```python
from build123d import *

# Parameters (mm, degrees)
F1_DEPTH = 3.175
F3_DEPTH = 12.7
F5_DEPTH = 12.7


with BuildPart() as f1:
    # F0 (on Top) → F1 (new body)
    with BuildSketch(Plane.XY):
        Polygon((-6.0333638393, 76.2), (-12.7, 0), (12.7, 0), (6.0333638393, 76.2), align=None)
    extrude(amount=-F1_DEPTH)

    # F2 (on face) → F3 (join)
    with BuildSketch(Plane.XY):
        Polygon((-2.8583638393, 76.2), (-6.0333638393, 76.2), (-12.7, 0), (-9.525, 0), align=None)
        Polygon((12.7, 0), (6.0333638393, 76.2), (2.8583638393, 76.2), (9.525, 0), align=None)
    extrude(amount=F3_DEPTH)

    # F4 (on face) → F5 (cut, through all)
    with BuildSketch(Plane.XY.offset(12.7)):
        Polygon((0, 15.875), (-11.3111174665, 15.875), (-12.4222234933, 3.175), (0, 3.175), align=None)
    extrude(amount=-F5_DEPTH, mode=Mode.SUBTRACT)


solid = f1.part
```
Build history of the part. All positions in model axes, mm. A direction names the side the tool comes from. Coordinates: 2 decimals unless noted, no trailing zeros. Write each loop counter-clockwise with the first axis right and the second up, starting at its lowest first coordinate (ties: lowest second). Pieces come first, ordered by that corner, then holes.
1. Band-saw the part on B-B, the plane y = 68.5. Give the cut face in (x, z) (3 decimals), and give its area (3 significant figures).
Answer block:
outline: (-6.707, -3.175) - (6.707, -3.175) - (6.707, 12.7) - (3.532, 12.7) - (3.532, 0) - (-3.532, 0) - (-3.532, 12.7) - (-6.707, 12.7) - close
area: 123 mm2
2. Band-saw the part on D-D, the plane z = -2. Give the cut face in (x, y), and give its area (3 significant figures).
Answer block:
outline: (-12.7, 0) - (12.7, 0) - (6.03, 76.2) - (-6.03, 76.2) - close
area: 1,430 mm2
3. Drop flat-ended pins along their axis: pin 1 (5 mm diameter, centred on y = 59.5, z = 5.5, fed in from -X); pin 2 (5 mm diameter, centred on x = -1.5, y = 22.5, fed in from +Z); pin 3 (5 mm diameter, centred on y = 66, z = 0.5, fed in from +X). Give the stop position or say it passes through.
Answer block:
pin 1: stops at x = -7.71
pin 2: stops at z = 0
pin 3: stops at x = 7.14
4. Drill centre lines: probe 1 along Z at (x, y) = (1.5, 64.5) (3 decimals); probe 2 along X at (y, z) = (55, 5); probe 3 along X at (y, z) = (68.5, 2.25). Where is each one in solid material? Low to high.
Answer block:
probe 1: z = -3.175 to 0
probe 2: x = -7.89 to -4.71, 4.71 to 7.89
probe 3: x = -6.71 to -3.53, 3.53 to 6.71
5. Pull direction Y, two halves, no side cores. Call faces 4 (the flat face through (-10, 15.875, 6)), 5 (the flat face through (0, 0, -1)), 6 (the flat face through (0, 30, -3.175)): released by +Y, released by -Y, zero draft, split by the parting line, or undercut.
Answer block:
face 4: undercut
face 5: released by -Y
face 6: zero draft
6. Band-saw the part on C-C, the plane x = 0. Give the cut face in (y, z) (3 decimals).
Answer block:
outline: (0, -3.175) - (76.2, -3.175) - (76.2, 0) - (0, 0) - close
7. Band-saw the part on A-A, the plane z = 7. Give the cut face in (x, y) (3 decimals).
Answer block:
outline: (-12.7, 0) - (-9.525, 0) - (-9.247, 3.175) - (-12.422, 3.175) - close; (-11.311, 15.875) - (-8.136, 15.875) - (-2.858, 76.2) - (-6.033, 76.2) - close; (2.858, 76.2) - (9.525, 0) - (12.7, 0) - (6.033, 76.2) - close
8. 3-axis set-ups, long thin cutter, end or side, ignore diameter. For faces 1 (the flat face through (6.145, 38.633, 6.261)), 2 (the flat face through (-11, 2, 12.7)), 3 (the flat face through (-11, 3.175, 6)): which of +Z, -Z, +X, -X, +Y, -Y reach the whole face in a straight line?
Answer block:
face 1: +Z, -Y
face 2: +Z, +X, -X, +Y, -Y
face 3: +Z, -X
